Input: dimensioned drawing with shaded views. Units: mm. Origin: part minimum x, y, z. A direction names the side the tool comes from. Coordinates: 2 decimals unless noted, no trailing zeros. Order: outer loops, then holes, each group sorted by start corner. A loop starts at its lowest first (then second) coordinate and runs counter-clockwise, first axis right, second up. Notation, with made-up numbers: (0.25, 23) -> (49.25, 23) arc R32 cw to (49.25, 62) -> close; hole circle Ø2 at (37, 23). An arc over 180 degrees is marked (long way). Answer in a Markdown table with one row per item. Add a question column.
1) Section query D-D on y = 64. Return the cut outline in (x, z) (1 decimal).
2) Section query A-A on z = 51.5. Return the cut outline in (x, y) (1 decimal), then the cut area to 3 significant figures.
3) Section query C-C on y = 30.5. Return the cut outline in (x, z) (1 decimal), then the cut area to 3 significant figures.
4) Set-up query: the marked faces 1, 2 and 3. Return all of +Z, -Z, +X, -X, +Y, -Y with unobstructed straight access to the full face (end or side cutting, diameter ignored); none if empty.
5) Section query B-B on y = 49. Return the cut outline in (x, z) (1 decimal), then the cut area to 3 significant figures.
6) Contact query for flat-ended pins moving along their axis: P1, Ø22.5, axis at y = 48, z = 27, coming from the -X side (1 decimal); P2, Ø5, axis at x = 89, z = 37, coming from the +Y side; P3, Ø9.5, axis at x = 20, z = 20.5, coming from the +Y side. Output: stop coordinate, or through.
7) Ray query, line 1 (Y direction, x = 198, z = 58.5); line 2 (X direction, y = 38, z = 55) (1 decimal); line 3 (X direction, y = 48, z = 14) (1 decimal). Return the intervals inside material, ascending. Write a range as from..to.
8) Pull-direction query (X, two-part tool) for the marked faces 4, 5, 6 and 7; classes: +X half, -X half, draft (parallel to the pull), parting line (faces both ways), or undercut.
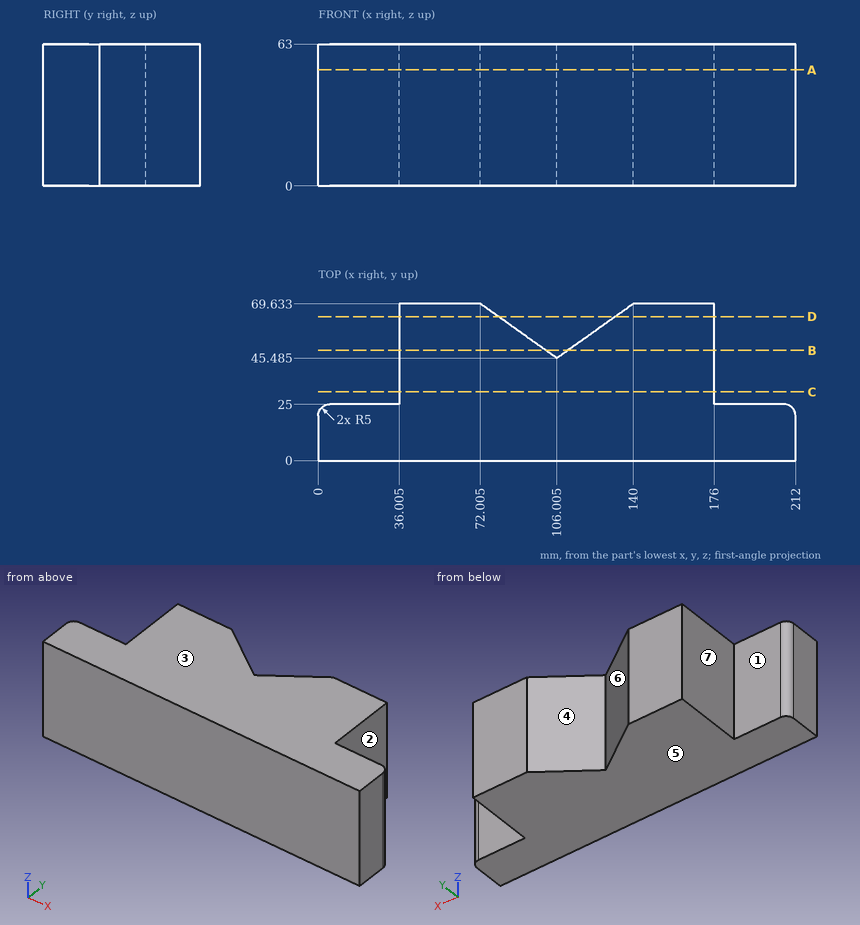
Result:
| question | item | result |
|---|---|---|
| 1 | outline | (36, 0) -> (79.9, 0) -> (79.9, 63) -> (36, 63) -> close; (132.1, 0) -> (176, 0) -> (176, 63) -> (132.1, 63) -> close |
| 2 | outline | (0, 0) -> (212, 0) -> (212, 20) arc R5 ccw to (207, 25) -> (176, 25) -> (176, 69.6) -> (140, 69.6) -> (106, 45.5) -> (72, 69.6) -> (36, 69.6) -> (36, 25) -> (5, 25) arc R5 ccw to (0, 20) -> close |
| 2 | area | 10,700 mm2 |
| 3 | outline | (36, 0) -> (176, 0) -> (176, 63) -> (36, 63) -> close |
| 3 | area | 8,820 mm2 |
| 4 | face 1 | +Z, -Z, -X, +Y |
| 4 | face 2 | +Z, -Z, +X, +Y |
| 4 | face 3 | +Z, +X, -X, +Y, -Y |
| 5 | outline | (36, 0) -> (101.1, 0) -> (101.1, 63) -> (36, 63) -> close; (111, 0) -> (176, 0) -> (176, 63) -> (111, 63) -> close |
| 5 | area | 8,200 mm2 |
| 6 | P1 | x = 36 |
| 6 | P2 | y = 59.34 |
| 6 | P3 | y = 25 |
| 7 | line 1 | 0..25 |
| 7 | line 2 | 36..176 |
| 7 | line 3 | 36..102.5, 109.5..176 |
| 8 | face 4 | undercut |
| 8 | face 5 | draft |
| 8 | face 6 | undercut |
| 8 | face 7 | -X half |
